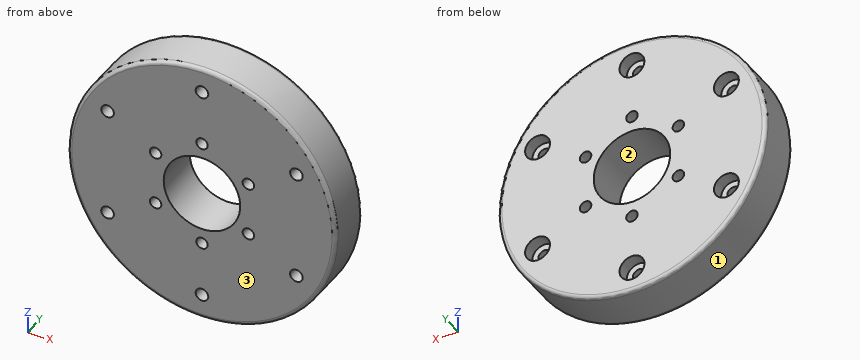
from build123d import *

# Parameters (mm, degrees)
SKETCH_1_R               = 35
EXTRUDE_1_DEPTH          = 12
HOLE_WIZARD_1_D          = 6.5
HOLE_WIZARD_1_DEPTH      = 3.3
PATTERN_CIRCULAR_1_COUNT = 6
HOLE_WIZARD_2_D          = 3.3
PATTERN_CIRCULAR_2_COUNT = 6
HOLE_WIZARD_3_D          = 3
PATTERN_CIRCULAR_3_COUNT = 6
FILLET_1_R               = 1
HOLE_WIZARD_4_D          = 20


with BuildPart() as part:
    # 草图1 → 凸台-拉伸1 (new body)
    with BuildSketch(Plane(origin=(0, 0, 0), x_dir=(1, 0, 0), z_dir=(0, 1, 0))):
        with Locations(Location((0, 0, 0), (0, 0, 270))):
            Circle(SKETCH_1_R)
    extrude(amount=EXTRUDE_1_DEPTH)

    # 孔1
    with Locations(Plane(origin=(0, 12, 0), x_dir=(1, 0, 0), z_dir=(0, 1, 0))):
        with Locations((0, 28.5)):
            hole_wizard_1 = Hole(HOLE_WIZARD_1_D / 2, depth=HOLE_WIZARD_1_DEPTH)

    # 阵列(圆周)1: 孔1 ×6 about axis
    pattern_circular_1_axis = Axis((0, 0, 0), (0, 1, 0))
    for i in range(1, PATTERN_CIRCULAR_1_COUNT):
        add(hole_wizard_1.rotate(pattern_circular_1_axis, i * 360 / PATTERN_CIRCULAR_1_COUNT), mode=Mode.SUBTRACT)

    # 孔2 (through all)
    with Locations(Plane(origin=(0, 8.7, 0), x_dir=(1, 0, 0), z_dir=(0, 1, 0))):
        with Locations((0, 28.5)):
            hole_wizard_2 = Hole(HOLE_WIZARD_2_D / 2)

    # 阵列(圆周)2: 孔2 ×6 about axis
    pattern_circular_2_axis = Axis((0, 0, 0), (0, 1, 0))
    for i in range(1, PATTERN_CIRCULAR_2_COUNT):
        add(hole_wizard_2.rotate(pattern_circular_2_axis, i * 360 / PATTERN_CIRCULAR_2_COUNT), mode=Mode.SUBTRACT)

    # 孔3 (through all)
    with Locations(Plane(origin=(0, 12, 0), x_dir=(1, 0, 0), z_dir=(0, 1, 0))):
        with Locations((0, 14)):
            hole_wizard_3 = Hole(HOLE_WIZARD_3_D / 2)

    # 阵列(圆周)3: 孔3 ×6 about axis
    pattern_circular_3_axis = Axis((0, 0, 0), (0, 1, 0))
    for i in range(1, PATTERN_CIRCULAR_3_COUNT):
        add(hole_wizard_3.rotate(pattern_circular_3_axis, i * 360 / PATTERN_CIRCULAR_3_COUNT), mode=Mode.SUBTRACT)

    # 圆角1
    fillet_1_edges = [part.edges().sort_by_distance(p)[0] for p in [
        (0, 0, -35),
        (0, 12, -35),
    ]]
    fillet(fillet_1_edges, radius=FILLET_1_R)

    # 孔4 (through all)
    with Locations(Plane(origin=(0, 12, 0), x_dir=(1, 0, 0), z_dir=(0, 1, 0))):
        with Locations((0, 0)):
            Hole(HOLE_WIZARD_4_D / 2)


solid = part.part
Model file for the job. Use its own axes, mm. Face numbers are marked on the shaded views. Give positions to 0.01 mm unless a question says otherwise; leave off trailing zeros. Use CSV: the item, a comma, the result in double quotes.
1. Drill centre lines: line 1 along X through (y, z) = (8.5, 8); line 2 along X through (y, z) = (5, -14.25); line 3 along Z through (x, y) = (-13.5, 1.5). Where is each one in solid material? Low to high. Write a range as from..to.
Outcome:
line 1,"-34.07..-13.24, -11.01..-6, 6..11.01, 13.24..34.07"
line 2,"-31.97..-26.33, -23.03..-1.48, 1.48..23.03, 26.33..31.97"
line 3,"-32.29..-7.6, -6.4..6.4, 7.6..32.29"
2. Drop flat-ended pins along their axis: pin 1 (2 mm diameter, centred on x = -23, z = 14.5, fed in from +Y); pin 2 (2 mm diameter, centred on x = -19.5, y = 8.5, fed in from -Z); pin 3 (6 mm diameter, centred on x = 18, y = 6.5, fed in from -Z). Give the stop position or say it passes through.
Outcome:
pin 1,"y = 8.7"
pin 2,"z = -29.71"
pin 3,"z = -31.62"
3. Band-saw the part on A-A, the plane y = 4.5. Count the separate pieces of the cut face and the enclosed holes in it, then the cut area to 3 significant figures.
Outcome:
separate pieces,"1"
enclosed holes,"13"
area,"3,440 mm²"
4. Mould opens along X. For the marked faces 1, 2 and 3 say: +X half, -X half, draft (parallel to the pull), parting line (faces both ways), or undercut.
Outcome:
face 1,"parting line"
face 2,"undercut"
face 3,"draft"
